Could you check a few things on this model? Use its own coordinates, in mm. Face numbers are marked on the shaded views. Round coordinates to 2 decimals unless told otherwise and drop trailing zeros. Loops run counter-clockwise (first coordinate to the right, second up) from the corner with the lowest first, then second, coordinate; pieces in that order, holes last. Notation, with made-up numbers: (-1, 75) - (16, 75) arc R13 ccw to (16, 91) - close; hole circle Ø11 at (-40, 68.5). An arc over 180 degrees is marked (long way). Use one line per item in the form item = value.
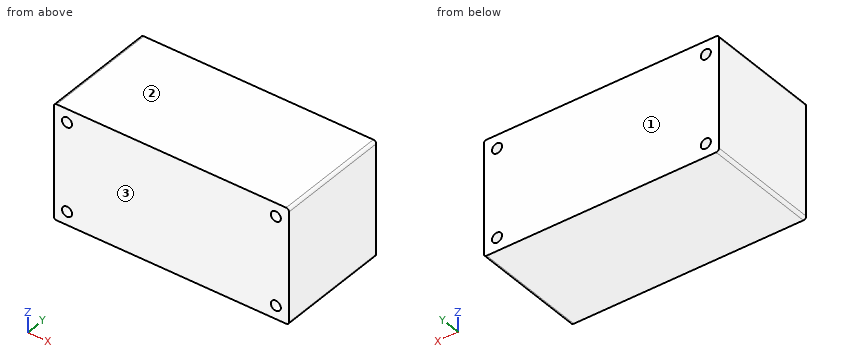
```python
from build123d import *

# Parameters (mm, degrees)
SKETCH2_W           = 41
SKETCH2_H           = 20
BOSS_EXTRUDE1_DEPTH = 20
FILLET1_R           = 0.5
SKETCH3_R           = 0.875
CUT_EXTRUDE1_DEPTH  = 21


with BuildPart() as part:
    # Sketch2 → Boss-Extrude1 (new body)
    with BuildSketch(Plane(origin=(0, 0, 0), x_dir=(1, 0, 0), z_dir=(0, 1, 0))):
        Rectangle(SKETCH2_W, SKETCH2_H)
    extrude(amount=BOSS_EXTRUDE1_DEPTH)

    # Fillet1
    fillet1_edges = [part.edges().sort_by_distance(p)[0] for p in [
        (20.5, 10, 10),
        (-20.5, 10, 10),
        (-20.5, 10, -10),
        (20.5, 10, -10),
    ]]
    fillet(fillet1_edges, radius=FILLET1_R)

    # Sketch3 → Cut-Extrude1 (cut, through all)
    with BuildSketch(Plane(origin=(0, 20, 0), x_dir=(1, 0, 0), z_dir=(0, 1, 0))):
        with Locations((18.190909091, 7.690909091)):
            Circle(SKETCH3_R)
        with Locations((18.190909091, -7.690909091)):
            Circle(SKETCH3_R)
        with Locations((-18.190909091, 7.690909091)):
            Circle(SKETCH3_R)
        with Locations((-18.190909091, -7.690909091)):
            Circle(SKETCH3_R)
    extrude(amount=-CUT_EXTRUDE1_DEPTH, mode=Mode.SUBTRACT)


solid = part.part
```
1. For P1, Ø2.5, axis at x = 18.19, z = -7.69, coming from the +Y side, with a flat end and sliding along its axis, tell me the tip position at first contact or that it passes through.
Solution:
P1 = 20
2. If we section it at A-A, the plane x = -18: Write out the boundary of the cut face in (y, z).
Solution:
outline = (0, -10) - (20, -10) - (20, -8.54) - (0, -8.54) - close; (0, -6.84) - (20, -6.84) - (20, 6.84) - (0, 6.84) - close; (0, 8.54) - (20, 8.54) - (20, 10) - (0, 10) - close
3. Please list where these lines run through material, in increasing order: line 1 along X through (y, z) = (3.25, 7.75); line 2 along X through (y, z) = (11.5, 7.5); line 3 along Z through (x, y) = (-18, 2.5).
Solution:
line_1 = -20.5 to -19.06, -17.32 to 17.32, 19.06 to 20.5
line_2 = -20.5 to -19.04, -17.34 to 17.34, 19.04 to 20.5
line_3 = -10 to -8.54, -6.84 to 6.84, 8.54 to 10
4. We'd pull the mould along Y, two halves only. Please class the marked faces 1, 2 and 3: +Y half, -Y half, draft (parallel to the pull), parting line (faces both ways), or undercut.
Solution:
face_1 = +Y half
face_2 = draft
face_3 = -Y half
